from build123d import *

# Parameters (mm, degrees)
F0_W     = 450
F0_H     = 45
F1_DEPTH = 7.5
F3_DEPTH = 20
F5_DEPTH = 20


with BuildPart() as f1:
    # F0 (on Top) → F1 (new body, symmetric)
    with BuildSketch(Plane.XY):
        Rectangle(F0_W, F0_H)
    extrude(amount=F1_DEPTH, both=True)

    # F2 (on face) → F3 (cut)
    with BuildSketch(Plane.YZ.offset(225)):
        with BuildLine():
            Line((22.5, 7.5), (6.6143782777, 7.5))
            ThreePointArc((6.6143782777, 7.5), (10, 0), (6.6143782777, -7.5))
            Line((6.6143782777, -7.5), (22.5, -7.5))
            Line((22.5, -7.5), (22.5, 7.5))
        make_face()
        with BuildLine():
            ThreePointArc((-6.6143782777, -7.5), (-10, 0), (-6.6143782777, 7.5))
            Line((-6.6143782777, 7.5), (-22.5, 7.5))
            Line((-22.5, 7.5), (-22.5, -7.5))
            Line((-22.5, -7.5), (-6.6143782777, -7.5))
        make_face()
    extrude(amount=-F3_DEPTH, mode=Mode.SUBTRACT)

    # F4 (on face) → F5 (cut)
    with BuildSketch(Plane(origin=(-225, 0, 0), x_dir=(0, -1, 0), z_dir=(-1, 0, 0))):
        with BuildLine():
            Line((22.5, 7.5), (6.6143782777, 7.5))
            ThreePointArc((6.6143782777, 7.5), (10, 0), (6.6143782777, -7.5))
            Line((6.6143782777, -7.5), (22.5, -7.5))
            Line((22.5, -7.5), (22.5, 7.5))
        make_face()
        with BuildLine():
            ThreePointArc((-6.6143782777, -7.5), (-10, 0), (-6.6143782777, 7.5))
            Line((-6.6143782777, 7.5), (-22.5, 7.5))
            Line((-22.5, 7.5), (-22.5, -7.5))
            Line((-22.5, -7.5), (-6.6143782777, -7.5))
        make_face()
    extrude(amount=-F5_DEPTH, mode=Mode.SUBTRACT)


solid = f1.part
Verification items for the finished model (mm, model axes). A direction names the side the tool comes from. Coordinates: 2 decimals unless noted, no trailing zeros. Order: outer loops, then holes, each group sorted by start corner. A loop starts at its lowest first (then second) coordinate and runs counter-clockwise, first axis right, second up. Notation, with made-up numbers: M 54.25,83 L 58.25,83 A18 ccw 58.25,100 Z; hole C 13,24.5 d11. An arc over 180 degrees is marked long. Return JSON: item names as keys, results as strings.
1) Thickness scan on L1, parallel to X at y = 18, z = 1. Record the ranges inside material, lowest first. Write a range as [from, to].
Answer list:
{"L1": "[-205, 205]"}
2) Cross-section at A-A, the plane z = -1. Record the boundary of the cut face in (x, y).
Answer list:
{"outline": "M -225,-9.95 L -205,-9.95 L -205,-22.5 L 205,-22.5 L 205,-9.95 L 225,-9.95 L 225,9.95 L 205,9.95 L 205,22.5 L -205,22.5 L -205,9.95 L -225,9.95 Z"}
3) Gauge pin test, flat ends, axial feed: pin 1 (3 mm diameter, centred on y = -18, z = -0.5, fed in from +X); pin 2 (7.5 mm diameter, centred on y = -17, z = 0.5, fed in from -X). Record the tip position at first contact, or that the pin passes through.
Answer list:
{"pin 1": "x = 205", "pin 2": "x = -205"}
4) Access from +Z, -Z, +X, -X, +Y, -Y to the whole of each face (thin tool, end or side, straight path). Record for faces 1 (the cylindrical face through (215, 10, 0)), 2 (the cylindrical face through (-215, -10, 0)), 3 (the cylindrical face through (-215, 10, 0)).
Answer list:
{"face 1": "+X, +Y", "face 2": "-X, -Y", "face 3": "-X, +Y"}
5) Cross-section at B-B, the plane y = 15.5. Record the boundary of the cut face in (x, z), and give its area (3 significant figures).
Answer list:
{"outline": "M -205,-7.5 L 205,-7.5 L 205,7.5 L -205,7.5 Z", "area": "6,150 mm2"}
